```python
from build123d import *

# Parameters (mm, degrees)
SKETCH2_W           = 5.1
SKETCH2_H           = 1.5875
SKETCH2_W_2         = 4.9
BOSS_EXTRUDE1_DEPTH = 1.5875


with BuildPart() as part:
    # Sketch2 → Boss-Extrude1 (new body)
    with BuildSketch(Plane.XY):
        Polygon((-19, -7.9), (-51, -7.9), (-51, -14.2125), (-45.9, -14.2125), (-23.9, -14.2125), (-19, -14.2125), align=None)
        with Locations((-48.45, -15.00625)):
            Rectangle(SKETCH2_W, SKETCH2_H)
        Polygon((-23.9, -1.5875), (-45.9, -1.5875), (-51, -1.5875), (-51, -7.9), (-19, -7.9), (-19, -1.5875), align=None)
        with Locations((-48.45, -0.79375)):
            Rectangle(SKETCH2_W, SKETCH2_H)
        with Locations((-21.45, -0.79375)):
            Rectangle(SKETCH2_W_2, SKETCH2_H)
        with Locations((-21.45, -15.00625)):
            Rectangle(SKETCH2_W_2, SKETCH2_H)
    extrude(amount=BOSS_EXTRUDE1_DEPTH)


solid = part.part
```
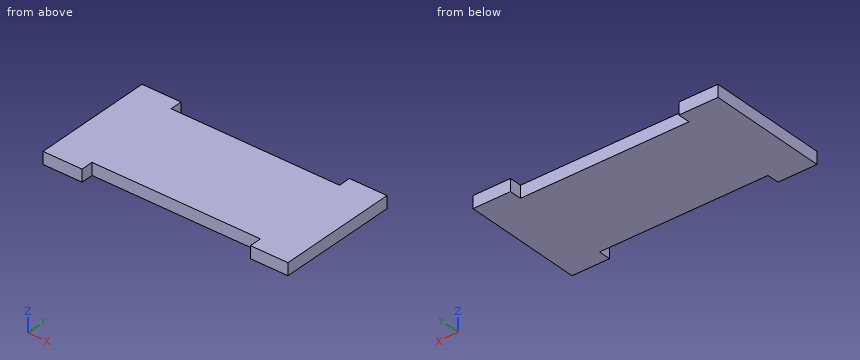
Work out the finished part from the listing and answer in its coordinate system (mm). Round coordinates to 2 decimals unless told otherwise and drop trailing zeros. Loops run counter-clockwise (first coordinate to the right, second up) from the corner with the lowest first, then second, coordinate; pieces in that order, holes last. Notation, with made-up numbers: (-8, -8.75) -> (32, -8.75) arc R13 cw to (32, 11.25) -> close; hole circle Ø10 at (-40, 12). An arc over 180 degrees is marked (long way). Write each question's results on one line, items separated by ' | '. Start each with the question number.
1. Section B-B (x = -40.5) is taken. Determine the outline of the cut face in (y, z).
2. Section A-A (z = 0.85) is taken. Determine the outline of the cut face in (x, y), plus the area to 3 significant figures.
3. Find the intervals of material crossed by probe 1 along X at (y, z) = (-14.5, 1.35); probe 2 along Y at (x, z) = (-44.5, 1.25), in increasing order. Write a range as from..to.
Evaluation:
1) outline: (-14.21, 0) -> (-1.59, 0) -> (-1.59, 1.59) -> (-14.21, 1.59) -> close
2) outline: (-51, -15.8) -> (-45.9, -15.8) -> (-45.9, -14.21) -> (-23.9, -14.21) -> (-23.9, -15.8) -> (-19, -15.8) -> (-19, 0) -> (-23.9, 0) -> (-23.9, -1.59) -> (-45.9, -1.59) -> (-45.9, 0) -> (-51, 0) -> close | area: 436 mm2
3) probe 1: x = -51..-45.9, -23.9..-19 | probe 2: y = -14.21..-1.59
